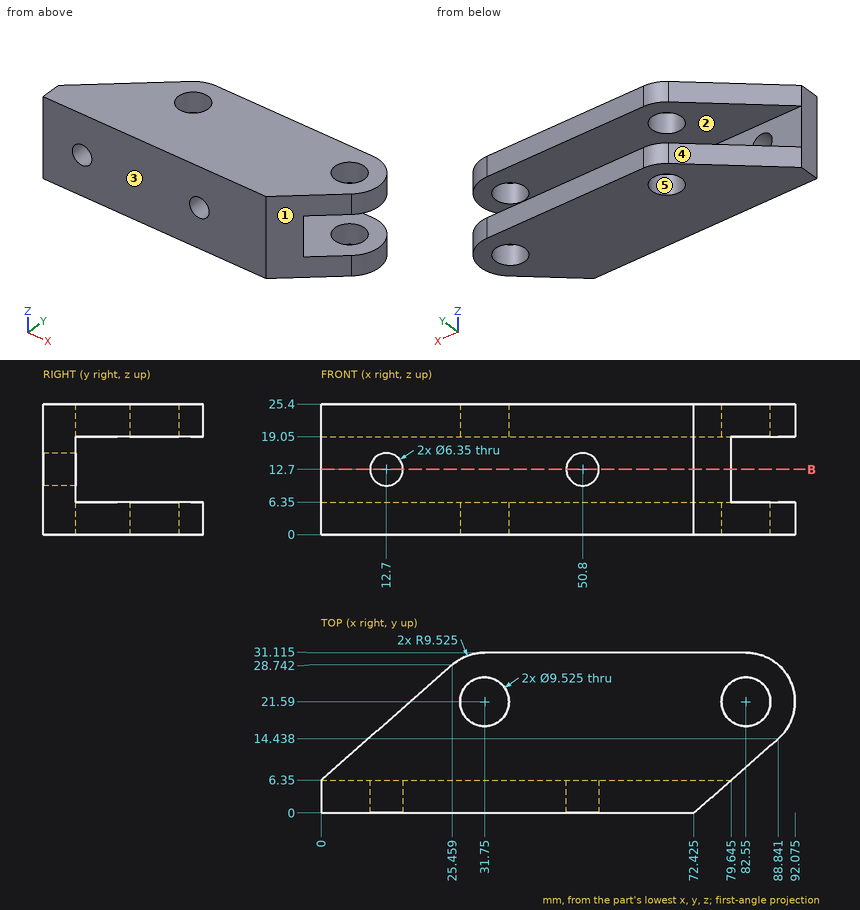
Study the drawing (mm; zero at the part's minimum x, y, z) and answer. A direction names the side the tool comes from. Coordinates: 2 decimals unless noted, no trailing zeros.
Q1. The mould has two halves that part along X. Classify the marked faces 3, 4 and 5: released by +X, released by -X, zero draft, split by the parting line, or undercut.
Returned:
face 3: zero draft
face 4: released by -X
face 5: undercut
Q2. Find the intervals of material crossed by line 1 along Z through (x, y) = (67, 29.5); line 2 along X through (y, z) = (1.5, 12.7) (1 decimal); line 3 along X through (y, z) = (21.59, 1.75) (1 decimal), in increasing order.
Returned:
line 1: z = 0 to 6.35, 19.05 to 25.4
line 2: x = 0 to 9.5, 15.9 to 47.6, 54 to 74.1
line 3: x = 17.3 to 27, 36.5 to 77.8, 87.3 to 92.1
Q3. Section B-B, the plane z = 12.7 is taken. Give the number of separate pieces and of enclosed holes in the cut face, then the cut area to 3 significant figures.
Returned:
separate pieces: 3
enclosed holes: 0
area: 402 mm2
Q4. Which of the six approach directions +Z, -Z, +X, -X, +Y, -Y give full straight-line access (tool end or side, diameter ignored) to the marked faces 1 and 2?
Returned:
face 1: +Z, -Z, +X, -Y
face 2: +X, -X, +Y
Q5. Given P1, Ø1, axis at y = 8.5, z = 9, coming from the -X side; P2, Ø7.5, axis at x = 50.8, z = 12.7, coming from the +Y side; P3, Ø5, axis at y = 20.5, z = 4.5, coming from the -X side (1 decimal), each flat-ended and moving along its own axis, determine where each tip first touches the part or whether it passes through.
Returned:
P1: passes through
P2: stops at y = 6.35
P3: stops at x = 13.2
